Geometry check sheet. Reference: drawing and pictorial views, mm from the part's lowest x, y, z. A direction names the side the tool comes from. Give positions to 0.01 mm unless a question says otherwise; leave off trailing zeros. Write each loop counter-clockwise with the first axis right and the second up, starting at its lowest first coordinate (ties: lowest second). Pieces come first, ordered by that corner, then holes. Notation, with made-up numbers: M -18,9 L 20,9 A19 ccw 20,14 Z; hole C 43.5,6.25 d5. An arc over 180 degrees is marked long. Write item = value, one per line. Start each with the question number.
1) Cross-section at D-D, the plane x = 18. Give the number of separate pieces and of enclosed holes in the cut face, plus the area to 3 significant figures.
2) Scan lines: line 1 along Y through (x, z) = (17, 18.75); line 2 along Y through (x, z) = (21, 39.5); line 3 along Z through (x, y) = (48, 11). Record each from-to range of solid material in increasing order. Write a range as [from, to].
3) Go/stop test with flat-tipped pins: pin 1 (3.5 mm diameter, centred on x = 18, z = 10, fed in from -Y); pin 2 (4 mm diameter, centred on y = 19.5, z = 10.5, fed in from -X); pin 3 (18 mm diameter, centred on x = 17, y = 25, fed in from -Z); pin 4 (10 mm diameter, centred on x = 41, y = 30.5, fed in from +Z). Record where each tip stops, or that it passes through.
4) Access from +Z, -Z, +X, -X, +Y, -Y to the whole of each face (thin tool, end or side, straight path). Record for the marked faces 1, 2 and 3.
5) Cross-section at A-A, the plane z = 21. Record the cut outline in (x, y), plus the area to 3 significant figures.
6) Mould release check, pull along X, two halves, no side actions. Record for the marked faces 4, 5, 6 and 7: released by +X, released by -X, zero draft, split by the parting line, or undercut.
7) Cross-section at C-C, the plane y = 29. Record the cut outline in (x, z).
8) Cross-section at B-B, the plane x = 62. Record the cut outline in (y, z).
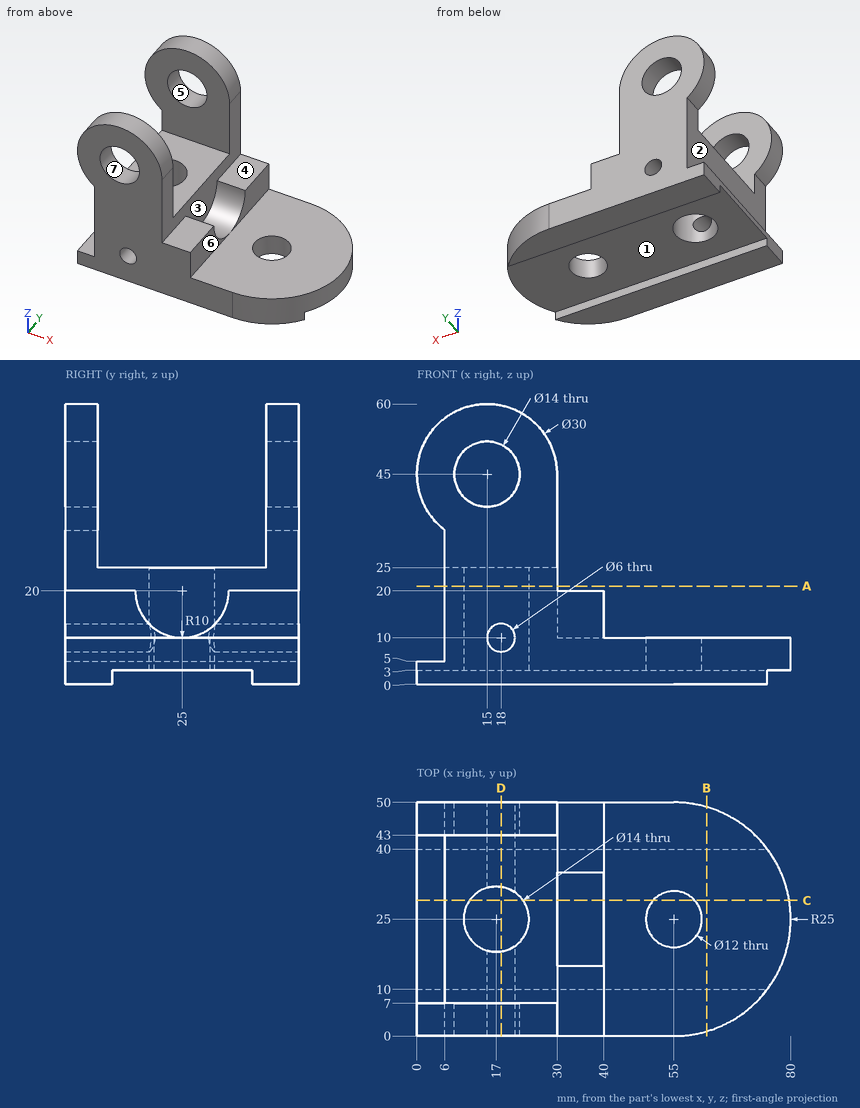
Reply:
q1.separate_pieces = 6
q1.enclosed_holes = 0
q1.area = 947 mm2
q2.line_1 = [0, 18], [32, 50]
q2.line_2 = [0, 7], [43, 50]
q2.line_3 = [3, 10]
q3.pin_1 = through
q3.pin_2 = 6
q3.pin_3 = 3
q3.pin_4 = 20
q4.face_1 = -Z, +X, -X
q4.face_2 = -X, +Y, -Y
q4.face_3 = +Z, +X
q5.outline = M 6,0 L 30,0 L 30,50 L 6,50 Z; hole C 17,25 d14
q5.area = 1,050 mm2
q6.face_4 = zero draft
q6.face_5 = undercut
q6.face_6 = released by +X
q6.face_7 = undercut
q7.outline = M 0,3 L 11.26,3 L 11.26,25 L 6,25 L 6,5 L 0,5 Z; M 22.74,3 L 50.53,3 L 50.53,10 L 40,10 L 40,10.83 L 30,10.83 L 30,25 L 22.74,25 Z; M 59.47,3 L 79.68,3 L 79.68,10 L 59.47,10 Z
q8.outline = M 1,0 L 10,0 L 10,3 L 40,3 L 40,0 L 49,0 L 49,10 L 1,10 Z
